Can you work these out from the drawing? Everything is in mm from the part's minimum corner. A direction names the side the tool comes from. Round coordinates to 2 decimals unless told otherwise and drop trailing zeros. Write each loop counter-clockwise with the first axis right and the second up, starting at its lowest first coordinate (ties: lowest second). Pieces come first, ordered by that corner, then holes. Notation, with made-up numbers: M 9,-15 L 13,-15 A21 cw 13,-7 Z; hole C -29.5,88 d11. An arc over 180 degrees is marked long. Use a Markdown table: item, result. Add a question column.
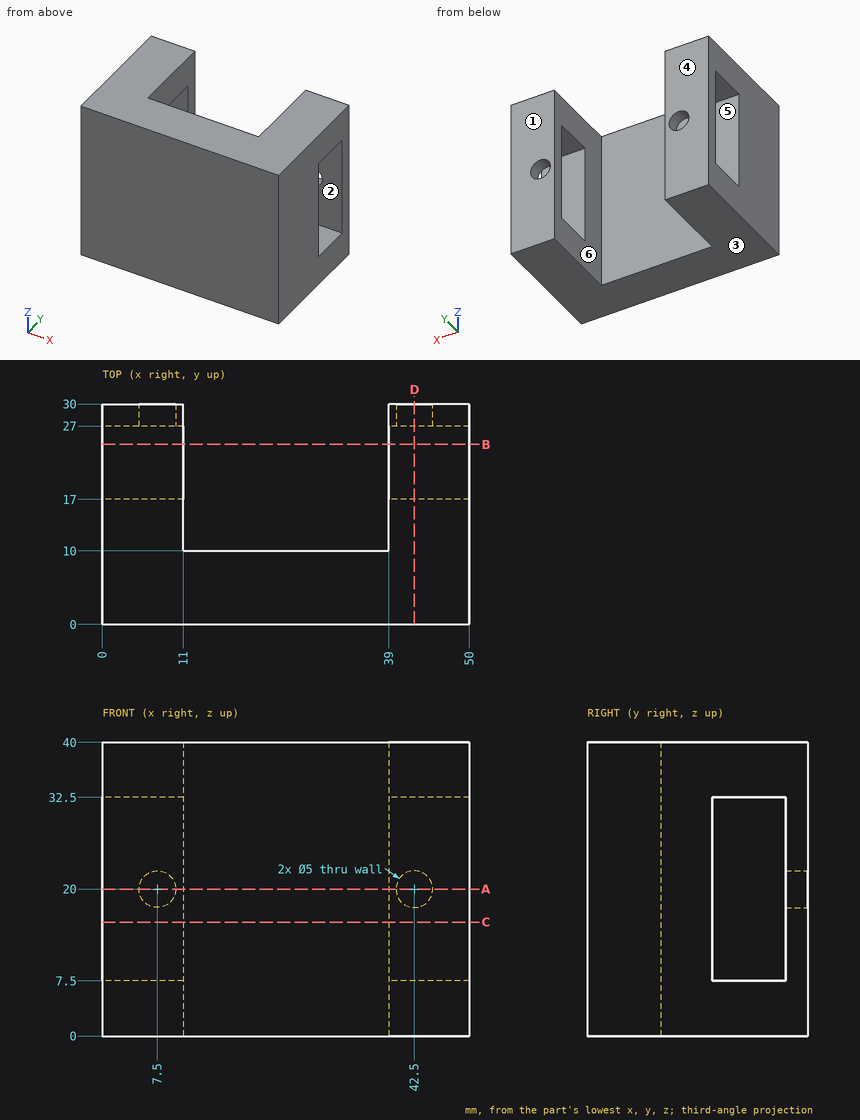
Item 1: For pin 1 Ø8 at (x, z) = (18, 24) entering from +Y; pin 2 Ø6 at (y, z) = (22.5, 27.5) entering from -X, each with a flat end and sliding along its axis, tell me the tip position at first contact or that it passes through.
Item 2: Imagine slicing it at A-A on z = 20. List the corners of the cut face in (x, y) for me, plus the area to 3 significant figures.
Item 3: Imagine slicing it at C-C on z = 15.5. List the corners of the cut face in (x, y) for me, plus the area to 3 significant figures.
Item 4: Imagine slicing it at D-D on x = 42.5. List the corners of the cut face in (y, z) for me.
Item 5: Imagine slicing it at B-B on y = 24.5. List the corners of the cut face in (x, z) for me, plus the area to 3 significant figures.
Item 6: On a 3-axis mill with a long thin cutter (end or side, diameter ignored), from which of +Z, -Z, +X, -X, +Y, -Y can I reach the whole of each face in a straight line? I mean the marked faces 4, 5 and 6. Say none if no direction works.
Item 7: I need wall thicknesses on probe 1 along X at (y, z) = (29.35, 20); probe 2 along X at (y, z) = (22.75, 34); probe 3 along Z at (x, y) = (7.5, 29.1). Which ranges of each line are inside material? Lowest first, please. Write a range as from..to.
Item 8: If we mould it in two halves opening along Y, with no side actions, what happens to the marked faces 1, 2 and 3? For each: +Y half, -Y half, draft (parallel to the pull), parting line (faces both ways), or undercut.
The answers:
| question | item | result |
|---|---|---|
| 1 | pin 1 | y = 10 |
| 1 | pin 2 | through |
| 2 | outline | M 0,0 L 50,0 L 50,17 L 39,17 L 39,10 L 11,10 L 11,17 L 0,17 Z; M 0,27 L 5,27 L 5,30 L 0,30 Z; M 10,27 L 11,27 L 11,30 L 10,30 Z; M 39,27 L 40,27 L 40,30 L 39,30 Z; M 45,27 L 50,27 L 50,30 L 45,30 Z |
| 2 | area | 690 mm² |
| 3 | outline | M 0,0 L 50,0 L 50,17 L 39,17 L 39,10 L 11,10 L 11,17 L 0,17 Z; M 0,27 L 11,27 L 11,30 L 0,30 Z; M 39,27 L 50,27 L 50,30 L 39,30 Z |
| 3 | area | 720 mm² |
| 4 | outline | M 0,0 L 30,0 L 30,17.5 L 27,17.5 L 27,7.5 L 17,7.5 L 17,32.5 L 27,32.5 L 27,22.5 L 30,22.5 L 30,40 L 0,40 Z |
| 5 | outline | M 0,0 L 11,0 L 11,7.5 L 0,7.5 Z; M 0,32.5 L 11,32.5 L 11,40 L 0,40 Z; M 39,0 L 50,0 L 50,7.5 L 39,7.5 Z; M 39,32.5 L 50,32.5 L 50,40 L 39,40 Z |
| 5 | area | 330 mm² |
| 6 | face 4 | +Z, -Z, +X, -X, +Y |
| 6 | face 5 | +X, -X |
| 6 | face 6 | +Z, -Z, +Y |
| 7 | probe 1 | 0..5, 10..11, 39..40, 45..50 |
| 7 | probe 2 | 0..11, 39..50 |
| 7 | probe 3 | 0..17.5, 22.5..40 |
| 8 | face 1 | +Y half |
| 8 | face 2 | undercut |
| 8 | face 3 | draft |
